Geometry check sheet. Reference: the model listing, model coordinates, mm. Face numbers are marked on the shaded views. Coordinates: 2 decimals unless noted, no trailing zeros. Write each loop counter-clockwise with the first axis right and the second up, starting at its lowest first coordinate (ties: lowest second). Pieces come first, ordered by that corner, then holes. Notation, with made-up numbers: M 52,63.5 L 87,63.5 A28 cw 87,82.5 Z; hole C 60,45.25 d9. An arc over 180 degrees is marked long. Put each result on its own line as item: value. Start each with the question number.
1) Mould release check, pull along Y, two halves, no side actions. Record for the marked faces 1 and 2: released by +Y, released by -Y, zero draft, split by the parting line, or undercut.
2) Cross-section at A-A on x = 0. Record the cut outline in (y, z) (3 decimals), plus the area to 3 significant figures.
3) Gauge pin test, flat ends, axial feed: pin 1 (1.5 mm diameter, centred on y = 10, z = 2.5, fed in from +X); pin 2 (1.5 mm diameter, centred on x = 10, z = 1.5, fed in from +Y); pin 3 (1 mm diameter, centred on y = 15, z = 0.5, fed in from -X); pin 4 (2 mm diameter, centred on x = 9, y = 5, fed in from +Z). Record the tip position at first contact, or that the pin passes through.
4) Cross-section at B-B on y = 5. Count the separate pieces of the cut face and the enclosed holes in it, plus the area to 3 significant figures.
5) Scan lines: line 1 along Y through (x, z) = (0, 0.1); line 2 along X through (y, z) = (4, 2.65); line 3 along Y through (x, z) = (-9, 1.4). Record each from-to range of solid material in increasing order.
from build123d import *

# Parameters (mm, degrees)
SKETCH1_R           = 25.5
BOSS_EXTRUDE1_DEPTH = 4
SKETCH3_R           = 24.5
SKETCH3_R_2         = 18.5
CUT_EXTRUDE1_DEPTH  = 1.675
FILLET1_R           = 1.5
FILLET2_R           = 2
SKETCH4_R           = 1.7
CUT_EXTRUDE2_DEPTH  = 4


with BuildPart() as part:
    # Sketch1 → Boss-Extrude1 (new body)
    with BuildSketch(Plane.XY):
        Circle(SKETCH1_R)
    extrude(amount=BOSS_EXTRUDE1_DEPTH)

    # Sketch3 → Cut-Extrude1 (cut)
    with BuildSketch(Plane(origin=(0, 0, 0), x_dir=(-1, 0, 0), z_dir=(0, 0, -1))):
        Circle(SKETCH3_R)
        Circle(SKETCH3_R_2, mode=Mode.SUBTRACT)
    extrude(amount=-CUT_EXTRUDE1_DEPTH, mode=Mode.SUBTRACT)

    # Fillet1
    fillet1_edges = [part.edges().sort_by_distance(p)[0] for p in [
        (24.5, 0, 1.675),
        (18.5, 0, 1.675),
    ]]
    fillet(fillet1_edges, radius=FILLET1_R)

    # Fillet2
    fillet2_edges = [part.edges().sort_by_distance(p)[0] for p in [
        (-25.5, 0, 4),
    ]]
    fillet(fillet2_edges, radius=FILLET2_R)

    # Sketch4 → Cut-Extrude2 (cut)
    with BuildSketch(Plane(origin=(0, 0, 0), x_dir=(-1, 0, 0), z_dir=(0, 0, -1))):
        with Locations((-9, 5)):
            Circle(SKETCH4_R)
        with Locations((9, 5)):
            Circle(SKETCH4_R)
    extrude(amount=-CUT_EXTRUDE2_DEPTH, mode=Mode.SUBTRACT)


solid = part.part
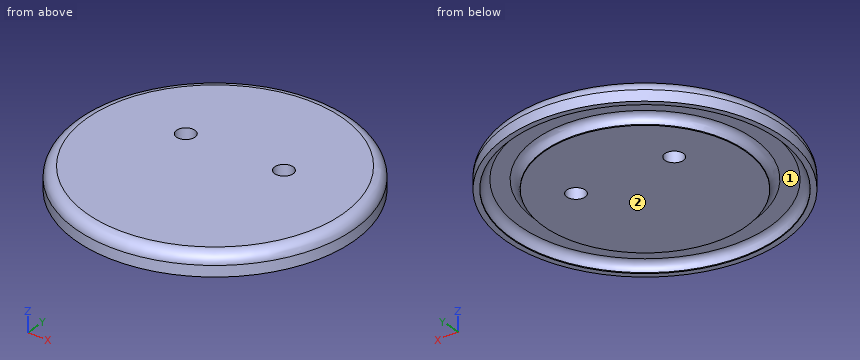
Answer key:
1. face 1: undercut
1. face 2: zero draft
2. outline: M -25.5,0 L -24.5,0 L -24.5,0.175 A1.5 cw -23,1.675 L -20,1.675 A1.5 cw -18.5,0.175 L -18.5,0 L 18.5,0 L 18.5,0.175 A1.5 cw 20,1.675 L 23,1.675 A1.5 cw 24.5,0.175 L 24.5,0 L 25.5,0 L 25.5,2 A2 ccw 23.5,4 L -23.5,4 A2 ccw -25.5,2 Z
2. area: 184 mm²
3. pin 1: stops at x = 23.73
3. pin 2: stops at y = 23.76
3. pin 3: stops at x = -20.98
3. pin 4: passes through
4. separate pieces: 3
4. enclosed holes: 0
4. area: 152 mm²
5. line 1: y = -25.5 to -24.5, -18.5 to 18.5, 24.5 to 25.5
5. line 2: x = -25.07 to -10.37, -7.63 to 7.63, 10.37 to 25.07
5. line 3: y = -23.86 to -22.1, -16.89 to 3.3, 6.7 to 16.89, 22.1 to 23.86
